```python
from build123d import *

# Parameters (mm, degrees)
SKETCH_1_R           = 1.5
EXTRUDE_1_DEPTH      = 4.2
FILLET_1_R           = 1.5
SKETCH_2_R           = 2
EXTRUDE_2_DEPTH      = 1
EXTRUDE_START        = 0.5
SKETCH_3_R           = 1.5
EXTRUDE_3_DEPTH      = 0.5
CHAMFER_1_SIZE       = 0.5
EXTRUDE_4_DEPTH      = 24.5
EXTRUDE_4_DEPTH_BACK = 0.5
SKETCH_4_R           = 0.25


with BuildPart() as part:
    # Эскиз1 → Бобышка-Вытянуть1 (new body)
    with BuildSketch(Plane.XY):
        Circle(SKETCH_1_R)
    extrude(amount=EXTRUDE_1_DEPTH)

    # Скругление1
    fillet_1_edges = [part.edges().sort_by_distance(p)[0] for p in [
        (-1.5, 0, 4.2),
    ]]
    fillet(fillet_1_edges, radius=FILLET_1_R)

    # Эскиз2 → Бобышка-Вытянуть2 (add)
    with BuildSketch(Plane(origin=(0, 0, 0), x_dir=(-1, 0, 0), z_dir=(0, 0, -1))):
        Circle(SKETCH_2_R)
    extrude(amount=EXTRUDE_2_DEPTH)

    # Эскиз3 → Бобышка-Вытянуть3 (add)
    with BuildSketch(Plane(origin=(0, 0, -1), x_dir=(-1, 0, 0), z_dir=(0, 0, -1)).offset(EXTRUDE_START)):
        Circle(SKETCH_3_R)
    extrude(amount=-EXTRUDE_3_DEPTH)

    # Фаска1
    chamfer_1_edges = [part.edges().sort_by_distance(p)[0] for p in [
        (1.5, 0, -1.5),
    ]]
    chamfer(chamfer_1_edges, length=CHAMFER_1_SIZE - 0.0001)  # a hair under: the kernel refuses the full size

    # Эскиз4 → Бобышка-Вытянуть4 (add, two sides: drawn at the far end of the back side and taken through both)
    with BuildSketch(Plane(origin=(0, 0, -1.5), x_dir=(-1, 0, 0), z_dir=(0, 0, -1)).offset(-EXTRUDE_4_DEPTH_BACK)):
        with Locations((0, 1.27)):
            Circle(SKETCH_4_R)
        with Locations((0, -1.27)):
            Circle(SKETCH_4_R)
    extrude(amount=EXTRUDE_4_DEPTH + EXTRUDE_4_DEPTH_BACK)


solid = part.part
```
The model under review builds one solid part; all positions refer to its coordinate system, in mm. A direction names the side the tool comes from. Round coordinates to 2 decimals unless told otherwise and drop trailing zeros. Loops run counter-clockwise (first coordinate to the right, second up) from the corner with the lowest first, then second, coordinate; pieces in that order, holes last.
Item 1: For faces 1 (the face through (0.434, -1.952, -0.493)), 2 (the face through (-1.5, 0.07, 1.33)), 3 (the face through (0, 0, -1.5)), list the 3-axis set-ups (+Z, -Z, +X, -X, +Y, -Y) from which the entire face can be reached by the end or side of a thin tool; tool diameter is ignored.
Determined:
face 1: +Z, -Z
face 2: +Z
face 3: -Z, +X, -X
Item 2: Clearance check with flat-ended pins moving along their axes: pin 1 Ø1.5 at (x, y) = (-1, 0.5) entering from +Z; pin 2 Ø1.5 at (y, z) = (-1.5, -21) entering from -X; pin 3 Ø1.6 at (x, y) = (0.5, 0) entering from -Z. State where each tip first meets the part, or that it passes through.
Determined:
pin 1: stops at z = 4.15
pin 2: stops at x = -0.25
pin 3: stops at z = -1.5
Item 3: Take a section at B-B (z = -10). Write out the cut boundary in (x, y).
Determined:
outline: circle Ø0.5 at (0, -1.27); circle Ø0.5 at (0, 1.27)
Item 4: For line 1 (Z direction, x = 0.75, y = 1.6); line 2 (Y direction, x = -0.2, z = -15); line 3 (Y direction, x = -0.1, z = -5.5), list the stretches that pass through material, from the lowest coordinate up.
Determined:
line 1: z = -1 to 0
line 2: y = -1.42 to -1.12, 1.12 to 1.42
line 3: y = -1.5 to -1.04, 1.04 to 1.5
Item 5: Take a section at C-C (z = 1). Write out the cut boundary in (x, y).
Determined:
outline: circle Ø3 at (0, 0)
